from build123d import *

# Parameters (mm, degrees)
F1_DEPTH  = 60
F3_DEPTH  = 42.4274068712
F4_R      = 3
F5_DEPTH  = 5
F6_R      = 6.1
F7_DEPTH  = 42.4274068712
F8_W      = 4
F8_H      = 30.587
F8_W_2    = 8
F8_H_2    = 34.8228137424
F9_DEPTH  = 34.831
F11_DEPTH = 12
F12_DEPTH = 20
F13_R     = 2.25
F14_DEPTH = 3
F15_W     = 20
F15_H     = 9
F16_DEPTH = 3
F17_R     = 1.15
F18_DEPTH = 25


with BuildPart() as f1:
    # F0 (on Front) → F1 (new body)
    with BuildSketch(Plane.XZ):
        Polygon((60, 60), (0, 0), (60, 0), align=None)
    extrude(amount=F1_DEPTH)

    # F2 (on face) → F3 (cut, through all)
    with BuildSketch(Plane(origin=(0, 0, 0), x_dir=(0, -1, 0), z_dir=(-0.7071067812, 0, 0.7071067812))):
        with BuildLine():
            Line((0, 84.8528137424), (0, 0))
            Line((0, 0), (26, 0))
            Line((26, 0), (26, 36.0857112298))
            ThreePointArc((26, 36.0857112298), (22.5, 42.43), (26, 48.7742887702))
            Line((26, 48.7742887702), (26, 84.8528137424))
            Line((26, 84.8528137424), (0, 84.8528137424))
        make_face()
        with BuildLine():
            Line((34, 84.8528137424), (34, 48.7742887702))
            ThreePointArc((34, 48.7742887702), (37.5, 42.43), (34, 36.0857112298))
            Line((34, 36.0857112298), (34, 0))
            Line((34, 0), (60, 0))
            Line((60, 0), (60, 84.8528137424))
            Line((60, 84.8528137424), (34, 84.8528137424))
        make_face()
    extrude(amount=-F3_DEPTH, mode=Mode.SUBTRACT)

    # F4 (on face) → F5 (join)
    with BuildSketch(Plane.XZ.offset(34)):
        with Locations((36.3863177288, 23.6187637227)):
            Circle(F4_R)
    extrude(amount=F5_DEPTH)

    # F6 (on face) → F7 (cut, through all)
    with BuildSketch(Plane(origin=(0, 0, 0), x_dir=(0, -1, 0), z_dir=(-0.7071067812, 0, 0.7071067812))):
        with Locations((30, 42.43)):
            Circle(F6_R)
    extrude(amount=-F7_DEPTH, mode=Mode.SUBTRACT)

    # F8 (on face) → F9 (cut, through all)
    with BuildSketch(Plane(origin=(0, 0, 0), x_dir=(0, -1, 0), z_dir=(-0.7071067812, 0, 0.7071067812))):
        with Locations((30, 19.5365)):
            Rectangle(F8_W, F8_H)
        with Locations((30, 67.4414068712)):
            Rectangle(F8_W_2, F8_H_2)
    extrude(amount=-F9_DEPTH, mode=Mode.SUBTRACT)

    # F10 (on face) → F11 (join)
    with BuildSketch(Plane.XZ.offset(34)):
        Polygon((3, 3), (0, 0), (51.032902229, 0), (48.032902229, 3), align=None)
    extrude(amount=F11_DEPTH)

    # F10 (on face) → F12 (join)
    with BuildSketch(Plane.XZ.offset(34)):
        Polygon((3, 3), (0, 0), (51.032902229, 0), (48.032902229, 3), align=None)
    extrude(amount=-F12_DEPTH)

    # F13 (on face) → F14 (cut, through all)
    with BuildSketch(Plane(origin=(0, 0, 0), x_dir=(1, 0, 0), z_dir=(0, 0, -1))):
        with Locations((10.5164511145, 40)):
            Circle(F13_R)
        with Locations((40.5164511145, 40)):
            Circle(F13_R)
        with Locations((40.5164511145, 20)):
            Circle(F13_R)
        with Locations((10.5164511145, 20)):
            Circle(F13_R)
    extrude(amount=-F14_DEPTH, mode=Mode.SUBTRACT)

    # F15 (on face) → F16 (cut, through all)
    with BuildSketch(Plane.XY.offset(3)):
        with Locations((25.2664511145, -21.5)):
            Rectangle(F15_W, F15_H)
        with Locations((25.2664511145, -38.5)):
            Rectangle(F15_W, F15_H)
    extrude(amount=-F16_DEPTH, mode=Mode.SUBTRACT)

    # F17 (on face) → F18 (cut)
    with BuildSketch(Plane.XZ.offset(34)):
        with Locations((36.3863177288, 23.6187637227)):
            Circle(F17_R)
    extrude(amount=F18_DEPTH, mode=Mode.SUBTRACT)


solid = f1.part
Design review of the part built by this model. Coordinates are the model's own, in mm. A direction names the side the tool comes from. Give positions to 0.01 mm unless a question says otherwise; leave off trailing zeros. Order: outer loops, then holes, each group sorted by start corner. A loop starts at its lowest first (then second) coordinate and runs counter-clockwise, first axis right, second up. Notation, with made-up numbers: (46, 61) - (50, 61) arc R15 ccw to (50, 90) - close; hole circle Ø10 at (66, 61.25). An arc over 180 degrees is marked (long way). Write item = value, one per line. Start each with the question number.
Q1. To check wall thickness, follow L1, parallel to Y at x = 22, z = 21; L2, parallel to X at y = -20, z = 2; L3, parallel to Z at x = 45, y = -44. State the ranges of each line that lie inside material, in increasing order. Write a range as from..to.
Q2. We need section B-B on x = 14.5. State the section outline as (y, z) points, plus the area to 3 significant figures.
Q3. Clearance check with flat-ended pins moving along their axes: pin 1 Ø3 at (x, y) = (31, -37.5) entering from -Z; pin 2 Ø8 at (y, z) = (-25, 25.5) entering from -X; pin 3 Ø5 at (y, z) = (-27.5, 9.5) entering from -X. State where each tip first meets the part, or that it passes through.
Q4. We need section C-C on x = 28. State how many separate pieces and enclosed holes the cut face has, plus the area to 3 significant figures.
Q5. Mouldability with a two-part tool opening along X and no side actions: class faces 5 (the face through (30, -30, 0)), 6 (the face through (35.266, -39, 2)), 7 (the face through (60, -29, 9)) as released by +X, released by -X, zero draft, split by the parting line, or undercut.
Q6. Tool access review of faces 1 (the face through (35.266, -22, 2)), 2 (the face through (25, -26, 8)), 3 (the face through (15.266, -39, 2)), 4 (the face through (35.237, -37.474, 23.669)): name each direction out of +Z, -Z, +X, -X, +Y, -Y from which nothing blocks a thin tool from reaching the whole face with its end or side.
Q7. We need section D-D on x = 7.5. State the section outline as (y, z) points, plus the area to 3 significant figures.
Q8. We need section A-A on y = -40. State the section outline as (x, z) points, plus the area to 3 significant figures.
Working result:
q1.L1 = -34..-32, -28..-26
q1.L2 = 2..8.27, 12.77..15.27, 35.27..38.27, 42.77..49.03
q1.L3 = 0..3
q2.outline = (-46, 0) - (-14, 0) - (-14, 3) - (-26, 3) - (-26, 14.5) - (-28, 14.5) - (-28, 3) - (-32, 3) - (-32, 14.5) - (-34, 14.5) - (-34, 3) - (-46, 3) - close
q2.area = 142 mm²
q3.pin_1 = 22.28
q3.pin_2 = 21.63
q3.pin_3 = 7
q4.separate_pieces = 3
q4.enclosed_holes = 1
q4.area = 151 mm²
q5.face_5 = zero draft
q5.face_6 = undercut
q5.face_7 = released by +X
q6.face_1 = -Z
q6.face_2 = none
q6.face_3 = +Z, -Z
q6.face_4 = -Y
q7.outline = (-46, 0) - (-14, 0) - (-14, 3) - (-26, 3) - (-26, 7.5) - (-28, 7.5) - (-28, 3) - (-32, 3) - (-32, 7.5) - (-34, 7.5) - (-34, 3) - (-46, 3) - close
q7.area = 114 mm²
q8.outline = (0, 0) - (8.27, 0) - (8.27, 3) - (3, 3) - close; (12.77, 0) - (15.27, 0) - (15.27, 3) - (12.77, 3) - close; (35.27, 0) - (38.27, 0) - (38.27, 3) - (35.27, 3) - close; (42.77, 0) - (51.03, 0) - (48.03, 3) - (42.77, 3) - close
q8.area = 57.1 mm²
